```python
from build123d import *

# Parameters (mm, degrees)
SKETCH1_R           = 2.2
BOSS_EXTRUDE1_DEPTH = 2.2
SKETCH2_R           = 2.225
CUT_EXTRUDE1_DEPTH  = 235.422353883


with BuildPart() as part:
    # Sketch1 → Boss-Extrude1 (new body)
    with BuildSketch(Plane(origin=(0, 0, 0), x_dir=(1, 0, 0), z_dir=(0, 1, 0))):
        Polygon((84, 207), (72, 194), (0, 194), (-72, 194), (-84, 207), (-110, 207), (-110, 181), (-97, 169), (-97, 97), (-97, 25), (-110, 13), (-110, -13), (-84, -13), (-72, 0), (0, 0), (72, 0), (84, -13), (110, -13), (110, 13), (97, 25), (97, 97), (97, 169), (110, 181), (110, 207), align=None)
        with Locations(Location((104.3, 201.3, 0), (0, 0, 270))):
            Circle(SKETCH1_R, mode=Mode.SUBTRACT)
        with Locations(Location((-104.3, 201.3, 0), (0, 0, 270))):
            Circle(SKETCH1_R, mode=Mode.SUBTRACT)
        with Locations(Location((-104.3, -7.3, 0), (0, 0, 270))):
            Circle(SKETCH1_R, mode=Mode.SUBTRACT)
        with Locations(Location((104.3, -7.3, 0), (0, 0, 270))):
            Circle(SKETCH1_R, mode=Mode.SUBTRACT)
    extrude(amount=BOSS_EXTRUDE1_DEPTH)

    # Sketch2 → Cut-Extrude1 (cut, through all)
    with BuildSketch(Plane(origin=(0, 2.2, 0), x_dir=(1, 0, 0), z_dir=(0, 1, 0))):
        with Locations(Location((-54.025, 179.025, 0), (0, 0, 270))):
            Circle(SKETCH2_R)
        with Locations(Location((-36.025, 179.025, 0), (0, 0, 270))):
            Circle(SKETCH2_R)
        with Locations(Location((-54.025, 155.025, 0), (0, 0, 270))):
            Circle(SKETCH2_R)
        with Locations(Location((-36.025, 155.025, 0), (0, 0, 270))):
            Circle(SKETCH2_R)
        with Locations(Location((36.025, 155.025, 0), (0, 0, 90))):
            Circle(SKETCH2_R)
        with Locations(Location((54.025, 155.025, 0), (0, 0, 90))):
            Circle(SKETCH2_R)
        with Locations(Location((36.025, 179.025, 0), (0, 0, 90))):
            Circle(SKETCH2_R)
        with Locations(Location((54.025, 179.025, 0), (0, 0, 90))):
            Circle(SKETCH2_R)
    extrude(amount=-CUT_EXTRUDE1_DEPTH, mode=Mode.SUBTRACT)


solid = part.part
```
Verification items for the finished model (mm, model axes). A direction names the side the tool comes from. Round coordinates to 2 decimals unless told otherwise and drop trailing zeros. Write each loop counter-clockwise with the first axis right and the second up, starting at its lowest first coordinate (ties: lowest second). Pieces come first, ordered by that corner, then holes.
1. Section check B-B on x = -24.5. Enter the section's corners in (y, z).
2. Section check C-C on z = -132. Enter the section's corners in (x, y), plus the area to 3 significant figures.
3. Section check A-A on y = 0.6. State how many separate pieces and enclosed holes the cut face has, plus the area to 3 significant figures.
4. Scan lines: L1, parallel to X at y = 1.1, z = -201.3; L2, parallel to X at y = 0.2, z = -154; L3, parallel to X at y = 0.6, z = -180 (3 decimals). Record each from-to range of solid material in increasing order.
5. Access from +Z, -Z, +X, -X, +Y, -Y to the whole of each face (thin tool, end or side, straight path). Record for faces 1 (the flat face through (77.916, 1.085, 6.409)), 2 (the flat face through (103.591, 1.085, -18.916)), 3 (the flat face through (-103.409, 1.085, -19.084)), 4 (the flat face through (-77.916, 1.085, -200.409)).
6. Draft check along Z on faces 5 (the flat face through (-78.084, 1.085, 6.591)), 6 (the flat face through (-2, 2.2, -99)), 7 (the flat face through (103.409, 1.085, -174.916)). Enter one of: +Z half, -Z half, draft (parallel to the pull), parting line (faces both ways), or undercut.
7. Gauge pin test, flat ends, axial feed: P1, Ø0.7, axis at y = 0.5, z = -66, coming from the +X side; P2, Ø1, axis at y = 1.5, z = -19, coming from the -X side. Record the tip position at first contact, or that the pin passes through.
Answer:
1. outline: (0, -194) - (2.2, -194) - (2.2, 0) - (0, 0) - close
2. outline: (-97, 0) - (97, 0) - (97, 2.2) - (-97, 2.2) - close
2. area: 427 mm2
3. separate pieces: 1
3. enclosed holes: 12
3. area: 40,100 mm2
4. L1: x = -110 to -106.5, -102.1 to -78.74, 78.74 to 102.1, 106.5 to 110
4. L2: x = -97 to -56, -52.05 to -38, -34.05 to 34.05, 38 to 52.05, 56 to 97
4. L3: x = -108.917 to -56.025, -52.025 to -38.025, -34.025 to 34.025, 38.025 to 52.025, 56.025 to 108.917
5. face 1: +Z, +Y, -Y
5. face 2: +X, +Y, -Y
5. face 3: -X, +Y, -Y
5. face 4: -Z, +Y, -Y
6. face 5: +Z half
6. face 6: draft
6. face 7: undercut
7. P1: stops at x = 97
7. P2: stops at x = -104.04
